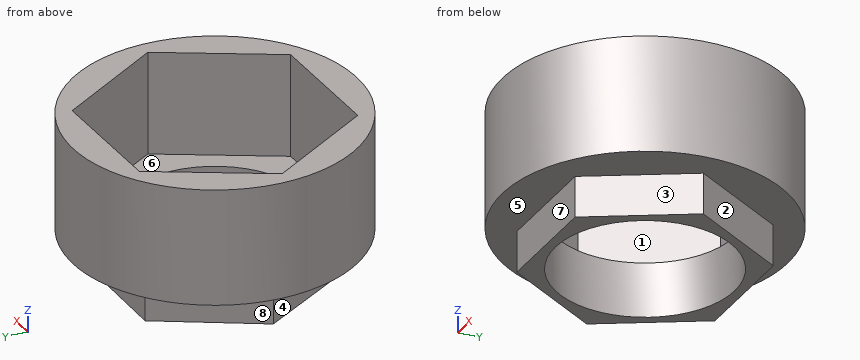
```python
from build123d import *

# Parameters (mm, degrees)
F1_DEPTH = 6
F2_R     = 20.7
F3_DEPTH = 2
F4_R     = 20.7
F5_DEPTH = 15
F6_R     = 13
F7_DEPTH = 25


with BuildPart() as f1:
    # F0 (on Top) → F1 (new body)
    with BuildSketch(Plane.XY):
        Polygon((8.29941, 14.375), (-8.29941, 14.375), (-16.59882, 0), (-8.29941, -14.375), (8.29941, -14.375), (16.59882, 0), align=None)
    extrude(amount=F1_DEPTH)

    # F2 (on face) → F3 (join)
    with BuildSketch(Plane.XY.offset(6)):
        Circle(F2_R)
    extrude(amount=F3_DEPTH)

    # F4 (on face) → F5 (join)
    with BuildSketch(Plane.XY.offset(8)):
        Circle(F4_R)
        Polygon((-9.523293, 15.831621), (8.948939, 16.163224), (18.472232, 0.331603), (9.523293, -15.831621), (-8.948939, -16.163224), (-18.472232, -0.331603), align=None, mode=Mode.SUBTRACT)
    extrude(amount=F5_DEPTH)

    # F6 (on face) → F7 (cut)
    with BuildSketch(Plane(origin=(0, 0, 0), x_dir=(1, 0, 0), z_dir=(0, 0, -1))):
        Circle(F6_R)
    extrude(amount=-F7_DEPTH, mode=Mode.SUBTRACT)


solid = f1.part
```
Verification items for the finished model (mm, model axes). Face numbers are marked on the shaded views. A direction names the side the tool comes from. Give positions to 0.01 mm unless a question says otherwise; leave off trailing zeros. Write each loop counter-clockwise with the first axis right and the second up, starting at its lowest first coordinate (ties: lowest second). Pieces come first, ordered by that corner, then holes. Notation, with made-up numbers: (39, 33) - (97, 33) arc R22 cw to (97, 57) - close; hole circle Ø6 at (64.5, 35). An arc over 180 degrees is marked (long way). Put each result on its own line as item: value.
Q1. Section check A-A on z = 2.5. Record the cut outline in (x, y) (3 decimals), and give its area (3 significant figures).
Result:
outline: (-16.599, 0) - (-8.299, -14.375) - (8.299, -14.375) - (16.599, 0) - (8.299, 14.375) - (-8.299, 14.375) - close; hole circle Ø26 at (0, 0)
area: 185 mm2
Q2. Depth check by flat-ended pin: P1, Ø6, axis at x = -10, y = 6, coming from the +Z side; P2, Ø8, axis at x = 0, z = 16.5, coming from the -Y side; P3, Ø3, axis at x = -7, y = 6.5, coming from the -Z side (3 decimals); P4, Ø1, axis at x = -10.5, z = 17, coming from the -Y side. Enter the tip coordinate at first touch or a pass-through.
Result:
P1: z = 8
P2: y = -20.7
P3: through
P4: y = -18.12
Q3. Set-up check for the marked faces 1, 2, 3, 4 and 5: record each of +Z, -Z, +X, -X, +Y, -Y from which the full face is reachable in a straight line by a thin tool's end or side.
Result:
face 1: +Z
face 2: -Z, +X, +Y
face 3: -Z, +X, -Y
face 4: -Z, -X, -Y
face 5: -Z
Q4. Mould release check, pull along Y, two halves, no side actions. Record for the marked faces 6, 7 and 8: released by +Y, released by -Y, zero draft, split by the parting line, or undercut.
Result:
face 6: undercut
face 7: released by -Y
face 8: released by +Y
Q5. Section check C-C on x = 12. Record the cut outline in (y, z), and give its area (3 significant figures).
Result:
outline: (-16.87, 6) - (-7.97, 6) - (-7.97, 0) - (-5, 0) - (-5, 8) - (-11.36, 8) - (-11.36, 23) - (-16.87, 23) - close; (5, 0) - (7.97, 0) - (7.97, 6) - (16.87, 6) - (16.87, 23) - (11.09, 23) - (11.09, 8) - (5, 8) - close
area: 252 mm2
Q6. Section check B-B on y = -1. Record the cut outline in (x, z).
Result:
outline: (-20.68, 6) - (-16.02, 6) - (-16.02, 0) - (-12.96, 0) - (-12.96, 8) - (-18.07, 8) - (-18.07, 23) - (-20.68, 23) - close; (12.96, 0) - (16.02, 0) - (16.02, 6) - (20.68, 6) - (20.68, 23) - (17.73, 23) - (17.73, 8) - (12.96, 8) - close
Q7. Scan lines: probe 1 along Y at (x, z) = (0, 4) (3 decimals); probe 2 along X at (y, z) = (0, 3.5); probe 3 along Y at (x, z) = (0, 6.25). Record each from-to range of solid material in increasing order. Write a range as from..to.
Result:
probe 1: -14.375..-13, 13..14.375
probe 2: -16.6..-13, 13..16.6
probe 3: -20.7..-13, 13..20.7
Q8. Section check D-D on z = 16.25. Record the cut outline in (x, y).
Result:
outline: circle Ø41.4 at (0, 0); hole (-18.47, -0.33) - (-8.95, -16.16) - (9.52, -15.83) - (18.47, 0.33) - (8.95, 16.16) - (-9.52, 15.83) - close
